Geometry check sheet. Reference: the model listing, model coordinates, mm. Round coordinates to 2 decimals unless told otherwise and drop trailing zeros. Loops run counter-clockwise (first coordinate to the right, second up) from the corner with the lowest first, then second, coordinate; pieces in that order, holes last. Notation, with made-up numbers: M 21,52.5 L 48,52.5 A8 cw 48,60.5 Z; hole C 16.25,31.25 d1. An arc over 180 degrees is marked long. Use one line per item in the form item = value. Start each with the question number.
1. Go/stop test with flat-tipped pins: pin 1 (10 mm diameter, centred on x = 2, y = 29, fed in from -Z); pin 2 (1 mm diameter, centred on x = 22.5, z = 2, fed in from -Y); pin 3 (1 mm diameter, centred on y = 4, z = 0.5, fed in from +X). Record where each tip stops, or that it passes through.
2. Cross-section at C-C (x = 12.5). Record the boundary of the cut face in (y, z), then the cut area to 3 significant figures.
3. Cross-section at B-B (y = -12.5). Record the boundary of the cut face in (x, z).
4. Material ranges on line 1 (Y direction, x = 5, z = 1.7) (3 decimals); line 2 (Y direction, x = 2.5, z = 2.7); line 3 (X direction, y = -16, z = 0.95), recorded low to high.
5. Cross-section at A-A (z = 1). Record the boundary of the cut face in (x, y), then the cut area to 3 significant figures.
6. Draft check along X on faces 1 (the flat face through (5.3, 6.4, 0)), 2 (the cylindrical face through (0, -15, 1)). Enter one of: pulls with the +X half, pulls with the -X half, needs draft (parallel to the pull), parting line crosses it, or undercut.
```python
from build123d import *

# Parameters (mm, degrees)
F0_R     = 11
F1_DEPTH = 3


with BuildPart() as f1:
    # F0 (on Top) → F1 (new body)
    with BuildSketch(Plane.XY):
        with BuildLine():
            ThreePointArc((0, 8), (-5.656854, -5.656854), (8, 0))
            ThreePointArc((8, 0), (5.656854, 5.656854), (0, 8))
        make_face()
        with BuildLine():
            ThreePointArc((11, 25), (-7.778175, 32.778175), (0, 14))
            ThreePointArc((0, 14), (7.778175, 17.221825), (11, 25))
        make_face()
        with BuildLine():
            ThreePointArc((8.291562, 12.5), (0, 40), (-8.291562, 12.5))
            ThreePointArc((-8.291562, 12.5), (-12.990381, 7.5), (-14.971099, 0.930703))
            ThreePointArc((-14.971099, 0.930703), (-34.641016, -20), (-6.679537, -13.430703))
            ThreePointArc((-6.679537, -13.430703), (0, -15), (6.679537, -13.430703))
            ThreePointArc((6.679537, -13.430703), (34.641016, -20), (14.971099, 0.930703))
            ThreePointArc((14.971099, 0.930703), (12.990381, 7.5), (8.291562, 12.5))
        make_face()
        with Locations((-21.650635, -12.5)):
            Circle(F0_R, mode=Mode.SUBTRACT)
        with Locations((21.650635, -12.5)):
            Circle(F0_R, mode=Mode.SUBTRACT)
        with BuildLine():
            ThreePointArc((0, 8), (5.656854, 5.656854), (8, 0))
            ThreePointArc((8, 0), (-5.656854, -5.656854), (0, 8))
        make_face(mode=Mode.SUBTRACT)
        with BuildLine():
            ThreePointArc((11, 25), (7.778175, 17.221825), (0, 14))
            ThreePointArc((0, 14), (-7.778175, 32.778175), (11, 25))
        make_face(mode=Mode.SUBTRACT)
    extrude(amount=F1_DEPTH)


solid = f1.part
```
Reported:
q1.pin_1 = through
q1.pin_2 = -27.5
q1.pin_3 = 14.59
q2.outline = M -24.39,0 L -18.6,0 L -18.6,3 L -24.39,3 Z; M -6.4,0 L 8.29,0 L 8.29,3 L -6.4,3 Z; M 16.71,0 L 33.29,0 L 33.29,3 L 16.71,3 Z
q2.area = 111 mm²
q3.outline = M -36.65,0 L -32.65,0 L -32.65,3 L -36.65,3 Z; M -10.65,0 L 10.65,0 L 10.65,3 L -10.65,3 Z; M 32.65,0 L 36.65,0 L 36.65,3 L 32.65,3 Z
q4.line_1 = -14.142 to -6.245, 6.245 to 15.202, 34.798 to 39.142
q4.line_2 = -14.79 to -7.6, 7.6 to 14.29, 35.71 to 39.79
q4.line_3 = -36.24 to -32.08, -11.22 to -7.06, 7.06 to 11.22, 32.08 to 36.24
q5.outline = M -14.97,0.93 A15 ccw long -6.68,-13.43 A15 ccw 6.68,-13.43 A15 ccw long 14.97,0.93 A15 ccw 8.29,12.5 A15 ccw long -8.29,12.5 A15 ccw Z; hole C -21.65,-12.5 d22; hole C 0,0 d16; hole M 0,14 A11 ccw 11,25 A11 ccw long Z; hole C 21.65,-12.5 d22
q5.area = 1,320 mm²
q6.face_1 = needs draft
q6.face_2 = undercut
